Read the model definition and answer for the solid it produces. Units are mm, in the model's axes. Face numbers are marked on the shaded views. A direction names the side the tool comes from. Coordinates: 2 decimals unless noted, no trailing zeros. Loops run counter-clockwise (first coordinate to the right, second up) from the corner with the lowest first, then second, coordinate; pieces in that order, holes last. Notation, with made-up numbers: (64.25, 44) -> (72.25, 44) arc R22 ccw to (72.25, 54) -> close; hole circle Ø10 at (0, -2). An arc over 180 degrees is marked (long way). Answer as CSV lines item,"result".
Autodesk Fusion 360 part; units mm, degrees
sketch "Spodek" plane through (0, 0, 0) normal (0, 0, 1) x (1, 0, 0)
  line L0 (0, 0) -> (61, 0)
  line L1 (61, 0) -> (61, 34)
  line L2 (61, 34) -> (0, 34)
  line L3 (0, 34) -> (0, 0)
  line L4 (-1, 35) -> (62, 35)
  line L5 (62, 35) -> (62, -1)
  line L6 (62, -1) -> (-1, -1)
  line L7 (-1, -1) -> (-1, 35)
  line L8 (-2.7, -2.7) -> (-2.7, 36.7) construction
  line L9 (63.7, 36.7) -> (-2.7, 36.7) construction
  line L10 (63.7, -2.7) -> (63.7, 36.7) construction
  line L11 (63.7, -2.7) -> (-2.7, -2.7) construction
  line L12 (-2.7, -2.7) -> (63.7, -2.7)
  line L13 (63.7, -2.7) -> (63.7, 36.7)
  line L14 (63.7, 36.7) -> (-2.7, 36.7)
  line L15 (-2.7, 36.7) -> (-2.7, -2.7)
  dimension "d1" = 61
  dimension "d2" = 34
  dimension "d3" = 63
  dimension "d4" = 36
  dimension "d5" = 1.7
  dimension "d6" = 1.7
  dimension "d7" = 1.7
  dimension "d8" = 1.7
sketch "TotoNevim" plane through (0, 0, 0) normal (0, 0, 1) x (1, 0, 0)
extrude "Extrude1" add sketch "Spodek" along normal blind 12 contours L12 L13 L14 L15 makes body 1
extrude "Extrude2" add sketch "Spodek" along normal blind 1.5 contours L0 L1 L2 L3 | L4 L5 L6 L7 bodies 1
sketch "Sketch3" plane through (0, 0, 1.5) normal (0, 0, 1) x (-1, 0, 0)
  line L0 (1, 1) -> (-62, 1)
  line L1 (-62, 1) -> (-62, -35)
  line L2 (-62, -35) -> (1, -35)
  line L3 (1, -35) -> (1, 1)
  line L4 (-59.78, -32.78) -> (-1.22, -32.78)
  line L5 (-1.22, -32.78) -> (-1.22, -1.22)
  line L6 (-1.22, -1.22) -> (-59.78, -1.22)
  line L7 (-59.78, -1.22) -> (-59.78, -32.78)
  line L8 (-61, 0) -> (-61, -34)
  line L9 (0, 0) -> (-61, 0)
  line L10 (0, -34) -> (0, 0)
  line L11 (-61, -34) -> (0, -34)
  dimension "d13" = 1.22
  dimension "d14" = 1.22
  dimension "d15" = 1.22
  dimension "d16" = 1.22
extrude "Extrude3" add sketch "Sketch3" along normal blind 1.8 contours L8 L9 L10 L11 bodies 1
extrude "Extrude4" add 1 faces at (20, -2.1333, 12) along direction (0, 0, 1) blind 5.243 on bodies 1 bodies 1
extrude "Extrude5" add 1 faces at (20, -2.1333, 17.243) along direction (0, 0, 1) blind 0.021 on bodies 1 bodies 1
sketch "Prurez1" plane through (-2.7, 0, 0) normal (-1, 0, 0) x (0, -1, 0)
  line L0 (-36.7, 0) -> (2.7, 0)
  line L1 (2.7, 0) -> (2.7, 17.264)
  line L2 (2.7, 17.264) -> (-36.7, 17.264)
  line L3 (-36.7, 17.264) -> (-36.7, 0)
  line L4 (-12, 3.3) -> (-12, 11) construction
  line L5 (0, 1.5) -> (0, 3.3) construction
  line L6 (-22, 11) -> (-22, 3.3) construction
  line L7 (-34, 3.3) -> (-34, 11) construction
  line L8 (-35, 1.5) -> (-35, 17.264) construction
  line L9 (-22, 11) -> (-12, 11) construction
  line L10 (-12, 11) -> (-12, 3.3) construction
  line L11 (-12, 3.3) -> (-22, 3.3) construction
  line L12 (-22, 3.3) -> (-22, 11) construction
  line L13 (-22, 11) -> (-12, 11)
  line L14 (-12, 11) -> (-12, 3.3)
  line L15 (-12, 3.3) -> (-22, 3.3)
  line L16 (-22, 3.3) -> (-22, 11)
  dimension "d23" = 7.7
  dimension "d24" = 12
  dimension "d25" = 12
  dimension "d26" = 1
extrude "Extrude6" cut sketch "Prurez1" against normal up to surface (66.4 mm away) contours L13 L14 L15 L16 bodies 1
sketch "Sketch5" plane through (0, 0, 17.264) normal (0, 0, 1) x (-1, 0, 0)
  line L0 (-62, 1) -> (1, 1)
  line L1 (1, 1) -> (1, -35)
  line L2 (1, -35) -> (-62, -35)
  line L3 (-62, -35) -> (-62, 1)
  line L4 (2.7, -36.7) -> (2.7, 2.7)
  line L5 (2.7, 2.7) -> (-63.7, 2.7)
  line L6 (-63.7, 2.7) -> (-63.7, -36.7)
  line L7 (-63.7, -36.7) -> (2.7, -36.7)
  line L8 (2.7, -36.7) -> (-63.7, -36.7)
  line L9 (-63.7, -36.7) -> (-63.7, 2.7)
  line L10 (-63.7, 2.7) -> (2.7, 2.7)
  line L11 (2.7, 2.7) -> (2.7, -36.7)
  line L12 (1, -35) -> (-62, -35)
  line L13 (-62, -35) -> (-62, 1)
  line L14 (-62, 1) -> (1, 1)
  line L15 (1, 1) -> (1, -35)
extrude "Extrude7" add sketch "Sketch5" along normal blind 3.7 bodies 1
sketch "Sketch6" plane through (-2.7, 0, 0) normal (-1, 0, 0) x (0, -1, 0)
  line L0 (-22, 3.3) -> (-22, 11)
  line L1 (-22, 11) -> (-12, 11)
  line L2 (-12, 11) -> (-12, 3.3)
  line L3 (-12, 3.3) -> (-22, 3.3)
  line L4 (-36.7, 0) -> (2.7, 0)
  line L5 (2.7, 0) -> (2.7, 20.964)
  line L6 (2.7, 20.964) -> (-36.7, 20.964)
  line L7 (-36.7, 20.964) -> (-36.7, 0)
  line L8 (-35, 17.264) -> (1.0001, 17.264)
  line L9 (1.0001, 17.264) -> (1.0001, 20.964)
  line L10 (1.0001, 20.964) -> (-35, 20.964)
  line L11 (-35, 20.964) -> (-35, 17.264)
  line L12 (-36.7, 17.264) -> (2.7, 17.264)
extrude "Extrude8" cut sketch "Sketch6" against normal up to surface (64.7 mm away) contours L6 L8 L9 L10 L11 L12 bodies 1
sketch "BokFront" plane through (0, -2.7, 0) normal (0, -1, 0) x (1, 0, 0)
  line L0 (-2.7, 0) -> (63.7, 0)
  line L1 (63.7, 0) -> (63.7, 20.964)
  line L2 (63.7, 20.964) -> (-2.7, 20.964)
  line L3 (-2.7, 20.964) -> (-2.7, 0)
  line L4 (-2.7, 20.964) -> (63.7, 20.964)
  line L5 (63.7, 20.964) -> (63.7, 17.264)
  line L6 (63.7, 17.264) -> (-2.7, 17.264)
  line L7 (-2.7, 17.264) -> (-2.7, 20.964)
  point P0 (63.7, 17.264)
sketch "BokRight" plane through (63.7, 0, 0) normal (1, 0, 0) x (0, 1, 0)
  line L0 (22, 11) -> (22, 3.3)
  line L1 (22, 3.3) -> (12, 3.3)
  line L2 (12, 3.3) -> (12, 11)
  line L3 (12, 11) -> (22, 11)
  line L4 (-2.7, 0) -> (36.7, 0)
  line L5 (36.7, 0) -> (36.7, 20.964)
  line L6 (36.7, 20.964) -> (-2.7, 20.964)
  line L7 (-2.7, 20.964) -> (-2.7, 0)
  line L8 (-2.7, 20.964) -> (36.7, 20.964)
  line L9 (36.7, 20.964) -> (36.7, 17.264)
  line L10 (36.7, 17.264) -> (-2.7, 17.264)
  line L11 (-2.7, 17.264) -> (-2.7, 20.964)
  point P0 (36.7, 17.264)
sketch "BokBack" plane through (0, 36.7, 0) normal (0, 1, 0) x (-1, 0, 0)
  line L0 (-63.7, 0) -> (2.7, 0)
  line L1 (2.7, 0) -> (2.7, 20.964)
  line L2 (2.7, 20.964) -> (-63.7, 20.964)
  line L3 (-63.7, 20.964) -> (-63.7, 0)
  line L4 (-63.7, 20.964) -> (2.7, 20.964)
  line L5 (2.7, 20.964) -> (2.7, 17.264)
  line L6 (2.7, 17.264) -> (-63.7, 17.264)
  line L7 (-63.7, 17.264) -> (-63.7, 20.964)
  point P0 (2.7, 17.264)
extrude "Extrude9" add sketch "BokBack" along normal blind 1.3 contours L1 L2 L3 L4 L5 L6 L7 bodies 1
extrude "Extrude10" add sketch "BokFront" along normal blind 1.3 contours L1 L2 L3 L4 L5 L6 L7 bodies 1
extrude "Extrude11" add sketch "BokRight" along normal blind 1.3 contours L5 L6 L7 L8 L9 L10 L11 bodies 1
extrude "Extrude12" add 1 faces at (63.7, 37.5667, 19.7307) along direction (1, 0, 0) blind 1.3 on bodies 1 bodies 1
extrude "Extrude13" add 1 faces at (63.7, -3.1333, 19.7307) along direction (1, 0, 0) blind 1.3 on bodies 1 bodies 1
sketch "Sketch10" plane through (-2.7, 0, 0) normal (-1, 0, 0) x (0, -1, 0)
  line L0 (-35, 17.264) -> (-35, 20.964)
  line L1 (-35, 20.964) -> (-38, 20.964)
  line L2 (-38, 20.964) -> (-38, 17.264)
  line L3 (-38, 17.264) -> (-36.7, 17.264)
  line L4 (-36.7, 17.264) -> (-36.7, 0)
  line L5 (-36.7, 0) -> (2.7, 0)
  line L6 (2.7, 0) -> (2.7, 17.264)
  line L7 (2.7, 17.264) -> (4, 17.264)
  line L8 (4, 17.264) -> (4, 20.964)
  line L9 (4, 20.964) -> (1.0001, 20.964)
  line L10 (1.0001, 20.964) -> (1.0001, 17.264)
  line L11 (1.0001, 17.264) -> (-35, 17.264)
  line L12 (-22, 3.3) -> (-22, 11)
  line L13 (-22, 11) -> (-12, 11)
  line L14 (-12, 11) -> (-12, 3.3)
  line L15 (-12, 3.3) -> (-22, 3.3)
  line L16 (4, 17.264) -> (2.7, 16)
  line L17 (-38, 17.264) -> (-36.7, 16)
extrude "Extrude14" add sketch "Sketch10" against normal up to surface (67.7 mm away) contours L3 L4 L17 | L6 L7 L16 bodies 1
sketch "Sketch11" plane through (0, -2.7, 0) normal (0, 1, 0) x (-1, 0, 0)
  line L0 (-63.7, 16) -> (-63.7, 17.264)
  line L1 (-63.7, 17.264) -> (-65, 17.264)
  line L2 (-65, 17.264) -> (-65, 16)
  line L3 (-65, 16) -> (-63.7, 16)
  line L4 (-65, 17.264) -> (-63.7, 16)
extrude "Extrude15" add sketch "Sketch11" along normal blind 39.4 contours L0 L1 L4 bodies 1
extrude "Extrude16" cut 1 faces at (64.5667, -2.7, 16.4213) along direction (0, -1, 0) blind 5.3 on bodies 1 bodies 1
extrude "Extrude17" cut 1 faces at (64.5667, 36.7, 16.4213) along direction (0, 1, 0) blind 1.9 on bodies 1 bodies 1
sketch "Sketch12" plane through (-2.7, 35.85, 19.114) normal (-1, 0, 0) x (0, -1, 0)
  line L0 (-0.85, 0) -> (0.85, 0)
  line L1 (0.85, 0) -> (0.85, -1.85)
  line L2 (0.85, -1.85) -> (-0.85, -1.85)
  line L3 (-0.85, -1.85) -> (-0.85, 0)
  line L4 (-0.85, 1.85) -> (-0.85, -19.114)
  line L5 (36.8501, -1.85) -> (38.55, -1.85)
  line L6 (38.55, -1.85) -> (38.55, 0)
  line L7 (38.55, 0) -> (36.8501, 0)
  line L8 (36.8501, 0) -> (36.8501, -1.85)
  line L9 (38.55, -19.114) -> (38.55, 1.85)
  point P0 (0.85, -1.85)
  point P1 (36.8501, -1.85)
extrude "Extrude18" cut sketch "Sketch12" against normal blind 64.7 bodies 1
sketch "Sketch13" plane through (62, 0, 0) normal (-1, 0, 0) x (0, -1, 0)
  line L0 (-35, 17.264) -> (-35, 1.5)
  line L1 (-35, 1.5) -> (1, 1.5)
  line L2 (1, 1.5) -> (1, 17.264)
  line L3 (1.0001, 17.264) -> (2.7, 17.264)
  line L4 (2.7, 17.264) -> (2.7, 19.114)
  line L5 (2.7, 19.114) -> (1.0001, 19.114)
  line L6 (1, 19.114) -> (1, 20.964)
  line L7 (1, 20.964) -> (-35, 20.964)
  line L8 (-35, 20.964) -> (-35, 19.114)
  line L9 (-35, 19.114) -> (-36.7, 19.114)
  line L10 (-36.7, 19.114) -> (-36.7, 17.264)
  line L11 (-36.7, 17.264) -> (-35, 17.264)
  line L12 (-22, 3.3) -> (-22, 11)
  line L13 (-22, 11) -> (-12, 11)
  line L14 (-12, 11) -> (-12, 3.3)
  line L15 (-12, 3.3) -> (-22, 3.3)
  line L16 (-36.7, 19.114) -> (2.7, 19.114)
  line L17 (2.7, 19.114) -> (2.7, 17.264)
  line L18 (2.7, 17.264) -> (-36.7, 17.264)
  line L19 (-36.7, 17.264) -> (-36.7, 19.114)
extrude "Extrude19" cut sketch "Sketch13" against normal blind 1.7 contours L3 L4 L5 L9 L10 L11 L16 L17 L18 L19 bodies 1
sketch "Sketch14" plane through (0, 0, 3.3) normal (0, 0, 1) x (-1, 0, 0)
  line L0 (0, -34) -> (0, 0)
  line L1 (0, 0) -> (-61, 0)
  line L2 (-61, 0) -> (-61, -34)
  line L3 (-61, -34) -> (0, -34)
  line L4 (-1.22, -1.22) -> (-1.22, -32.78)
  line L5 (-1.22, -32.78) -> (-59.78, -32.78)
  line L6 (-59.78, -32.78) -> (-59.78, -1.22)
  line L7 (-59.78, -1.22) -> (-1.22, -1.22)
  circle A0 centre (-58.6, -31.85) radius 1
  line L8 (-61, -17) -> (0, -17) construction
  circle A1 centre (-58.6, -2.15) radius 1
  line L9 (-30.5, -34) -> (-30.5, 0) construction
  circle A2 centre (-2.4, -31.85) radius 1
  circle A3 centre (-2.4, -2.15) radius 1
  point P0 (-58.6, -31.85)
  dimension "d55" = 2.15
  dimension "d56" = 2.4
  dimension "d57" = 2
extrude "Extrude20" add sketch "Sketch14" along normal blind 5 separate body contours L7 A3 | L5 A2 | L7 A1 | L5 A0 picked at (-2.3172, -1.2071) picked at (-2.278, -32.1598) picked at (-58.5172, -1.2071) picked at (-58.3551, -31.7867) makes body 2 at (59.2633, 32.5983, 6.6333) makes body 3 at (58.2716, 1.2054, 4.9667) makes body 4 at (3.0633, 32.5983, 6.6333) makes body 5 at (2.0716, 1.2054, 4.9667)
extrude "Extrude21" add 4 faces at (2.3172, 1.2071, 3.3) (2.278, 32.1598, 3.3) (58.3551, 31.7867, 3.3) (58.5172, 1.2071, 3.3) along direction (0, 0, -1) blind 2 on bodies 2 3 4 5 bodies 5 1 2 3 4
equation "d19 = 14 mm - 8.757 mm"
equation "d21 = 14 mm - 13.979 mm"
equation "d33 = 3 mm - 1.70 mm"
equation "d35 = 3 mm - 1.70 mm"
equation "d37 = 3 mm - 1.70 mm"
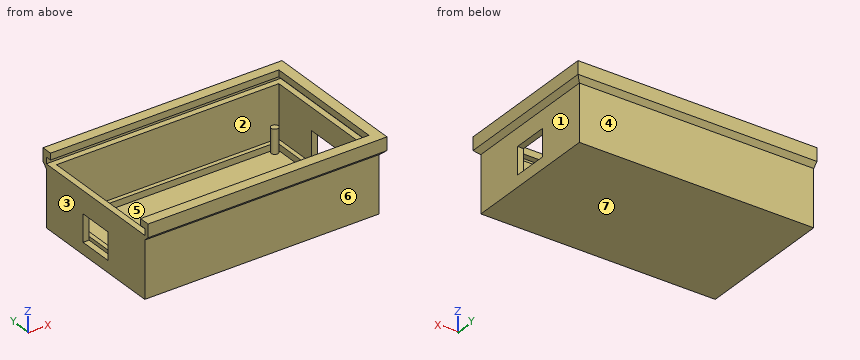
Q1. Given pin 1 Ø10 at (x, z) = (48, 3.5) entering from +Y; pin 2 Ø0.5 at (y, z) = (20.5, 2) entering from +X; pin 3 Ø0.8 at (x, z) = (-1.5, 9) entering from -Y, each flat-ended and moving along its own axis, determine where each tip first touches the part or whether it passes through.
Results:
pin 1,"stops at y = 36.7"
pin 2,"stops at x = 63.7"
pin 3,"stops at y = -2.7"
Q2. For the marked faces 1, 2 and 3, determine the directions among +Z, -Z, +X, -X, +Y, -Y from which every point of the face is accessible in a straight line to the end or side of a thin tool.
Results:
face 1,"-Z, +X, +Y, -Y"
face 2,"+Z"
face 3,"+Z, -Z, -X, +Y, -Y"
Q3. A cutting plane is placed at A-A, the plane z = 9. Write down the section's boundary in (x, y), and give its area (3 significant figures).
Results:
outline,"(-2.7, -2.7) -> (63.7, -2.7) -> (63.7, 12) -> (62, 12) -> (62, -1) -> (-1, -1) -> (-1, 12) -> (-2.7, 12) -> close; (-2.7, 22) -> (-1, 22) -> (-1, 35) -> (62, 35) -> (62, 22) -> (63.7, 22) -> (63.7, 36.7) -> (-2.7, 36.7) -> close"
area,"314 mm²"
Q4. A cutting plane is placed at C-C, the plane z = 13. Write down the section's boundary in (x, y).
Results:
outline,"(-2.7, -2.7) -> (63.7, -2.7) -> (63.7, 36.7) -> (-2.7, 36.7) -> close; hole (-1, -1) -> (62, -1) -> (62, 35) -> (-1, 35) -> close"
Q5. A cutting plane is placed at D-D, the plane x = 50. Write down the section's boundary in (y, z), and give its area (3 significant figures).
Results:
outline,"(-4, 17.26) -> (-2.7, 16) -> (-2.7, 0) -> (36.7, 0) -> (36.7, 16) -> (38, 17.26) -> (38, 20.96) -> (35, 20.96) -> (35, 19.11) -> (36.7, 19.11) -> (36.7, 17.26) -> (35, 17.26) -> (35, 1.5) -> (34, 1.5) -> (34, 3.3) -> (32.78, 3.3) -> (32.78, 1.5) -> (1.22, 1.5) -> (1.22, 3.3) -> (0, 3.3) -> (0, 1.5) -> (-1, 1.5) -> (-1, 17.26) -> (-2.7, 17.26) -> (-2.7, 19.11) -> (-1, 19.11) -> (-1, 20.96) -> (-4, 20.96) -> close"
area,"135 mm²"
Q6. A cutting plane is placed at B-B, the plane y = 13. Give the number of separate pieces and of enclosed holes in the cut face, and give its area (3 significant figures).
Results:
separate pieces,"3"
enclosed holes,"0"
area,"140 mm²"
Q7. Find the intervals of material crossed by probe 1 along X at (y, z) = (34, 13); probe 2 along Y at (x, z) = (52, 17.5); probe 3 along Z at (x, y) = (17, 36.5), in increasing order. Write a range as [from, to].
Results:
probe 1,"x = [-2.7, -1], [62, 63.7]"
probe 2,"y = [-4, -2.7], [36.7, 38]"
probe 3,"z = [0, 17.26], [19.11, 20.96]"
Q8. For a pull along Y with two mould halves and no side action, classify the marked faces 4, 5, 6 and 7 as pulls with the +Y half, pulls with the -Y half, needs draft (parallel to the pull), parting line crosses it, or undercut.
Results:
face 4,"pulls with the +Y half"
face 5,"undercut"
face 6,"pulls with the -Y half"
face 7,"needs draft"
